Autodesk Inventor part; units mm, degrees
ref_plane "YZ Plane" through (0, 0, 0) normal (1, 0, 0) x (0, 1, 0)
ref_plane "XZ Plane" through (0, 0, 0) normal (0, 1, 0) x (-1, 0, 0)
ref_plane "XY Plane" through (0, 0, 0) normal (0, 0, 1) x (1, 0, 0)
sketch "Esboço1" plane through (0, 0, 0) normal (0, 1, 0) x (-1, 0, 0)
  circle A0 centre (0, 0) radius 5
  dimension "d1" = 10
extrude "Extrusão1" add sketch "Esboço1" along normal blind 85
sketch "Esboço2" plane through (0, 0, 0) normal (0, -1, 0) x (1, 0, 0)
  circle A0 centre (0, 0) radius 5
hole "Furo1" at (0, 0, 0) direction (0, 1, 0) diameter 4.134 depth 14.2 tip angle 118
sketch "Esboço3" plane through (0, 85, 0) normal (0, 1, 0) x (1, 0, 0)
  circle A0 centre (0, 0) radius 5
hole "Furo2" at (0, 85, 0) direction (0, -1, 0) diameter 4.134 depth 14.2 tip angle 118
equation "\"Raio_vergadura\" = Espessura"
equation "\"Largura_alívio_de_vergadura\" = Espessura"
equation "\"Profundidade_alívio_de_vergadura\" = 0.5 * Espessura"
equation "\"Tamanho_alívio_de_dobra\" = 4 * Espessura"
equation "\"Remanescente_mínimo\" = 2 * Espessura"
equation "\"Raiodetransição\" = Raio_vergadura"
equation "\"Tamanho_de_raio_de_Jacobi\" = Raio_vergadura"
equation "\"TamanhoFolga\" = Espessura"
properties part number "Sustentação do motor" material "Latão, amarelo macio"
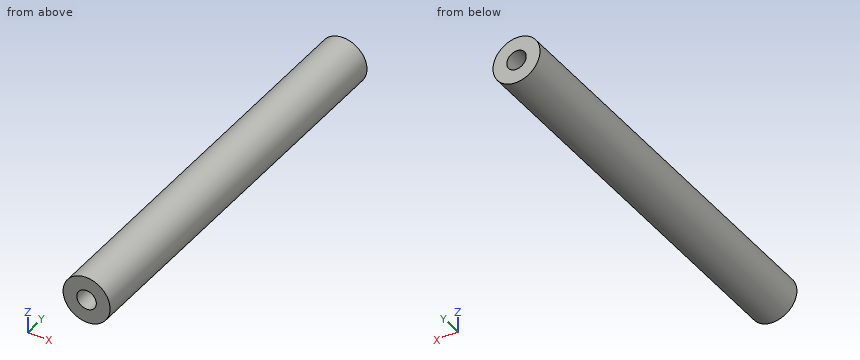
Can you work these out from the model? Positions are in its coordinate system, mm. Round coordinates to 2 decimals unless told otherwise and drop trailing zeros. Loops run counter-clockwise (first coordinate to the right, second up) from the corner with the lowest first, then second, coordinate; pieces in that order, holes last. Notation, with made-up numbers: (62.25, 68) -> (119.25, 68) arc R14 cw to (119.25, 93) -> close; hole circle Ø1 at (16, 17.5). An arc over 180 degrees is marked (long way). Answer in a Markdown table with one row per item.
Item 1: Will these pins go through, and if not, where does the flat tip stop? P1, Ø6, axis at y = 75.5, z = -0.5, coming from the -X side; P2, Ø3.5, axis at x = 0, z = 0, coming from the +Y side; P3, Ø2, axis at y = 31, z = -2.5, coming from the +X side; P4, Ø5, axis at x = 3.5, y = 34.5, coming from the -Z side.
Answer block:
| item | result |
|---|---|
| P1 | x = -5 |
| P2 | y = 70.61 |
| P3 | x = 4.77 |
| P4 | z = -4.9 |
Item 2: Suppose I cut it at C-C, the plane y = 64.5. List the corners of the cut face in (x, z) for me.
Answer block:
| item | result |
|---|---|
| outline | circle Ø10 at (0, 0) |
Item 3: Suppose I cut it at D-D, the plane z = -3.25. List the corners of the cut face in (x, y) for me, plus the area to 3 significant figures.
Answer block:
| item | result |
|---|---|
| outline | (-3.8, 0) -> (3.8, 0) -> (3.8, 85) -> (-3.8, 85) -> close |
| area | 646 mm² |
Item 4: If I drill on probe 1 along Z at (x, y) = (0, 76); probe 2 along X at (y, z) = (74.5, -0.75); probe 3 along Z at (x, y) = (1.25, 10.5), over which ranges is the centre line in solid material (lowest first)?
Answer block:
| item | result |
|---|---|
| probe 1 | -5 to -2.07, 2.07 to 5 |
| probe 2 | -4.94 to -1.93, 1.93 to 4.94 |
| probe 3 | -4.84 to -1.65, 1.65 to 4.84 |
Item 5: Suppose I cut it at B-B, the plane x = 4. List the corners of the cut face in (y, z) for me.
Answer block:
| item | result |
|---|---|
| outline | (0, -3) -> (85, -3) -> (85, 3) -> (0, 3) -> close |
Item 6: Suppose I cut it at A-A, the plane y = 8.5. List the corners of the cut face in (x, z) for me.
Answer block:
| item | result |
|---|---|
| outline | circle Ø10 at (0, 0); hole circle Ø4.13 at (0, 0) |
